Study the drawing (mm; zero at the part's minimum x, y, z) and answer. Coordinates: 2 decimals unless noted, no trailing zeros. Order: outer loops, then holes, each group sorted by start corner. A loop starts at its lowest first (then second) coordinate and runs counter-clockwise, first axis right, second up. Notation, with made-up numbers: M 40.5,65 L 63.5,65 A29 cw 63.5,94 Z; hole C 11,5 d5. An arc over 180 degrees is marked long. One line per item, written item: value. Start each with the question number.
Q1. The part is cut by section D-D on x = 6.5. Give the vertices of the cut face in (y, z), then the cut area to 3 significant figures.
Q2. The part is cut by section C-C on y = 26. Give the vertices of the cut face in (x, z), then the cut area to 3 significant figures.
Q3. The part is cut by section A-A on x = 25.8. Give the vertices of the cut face in (y, z).
Q4. Each of these flat-tipped pins is pushed along its axis until it touches: pin 1 Ø0.6 at (x, z) = (13.5, 2) entering from +Y; pin 2 Ø1.8 at (x, y) = (2, 2) entering from -Z; pin 3 Ø0.6 at (y, z) = (10, 2.5) entering from +X; pin 4 Ø3 at (x, y) = (25.8, 2) entering from +Z. Where does it stop, or does it pass through?
Q5. The part is cut by section B-B on z = 0.9. Give the vertices of the cut face in (x, y).
Q6. Straight lines are drawn through the part: line 1 along Y through (x, z) = (25.8, 0.8); line 2 along X through (y, z) = (12, 1.45); line 3 along Y through (x, z) = (26.25, 1.35). For each, find the intervals that lie inside material, in ascending order. Write a range as [from, to].
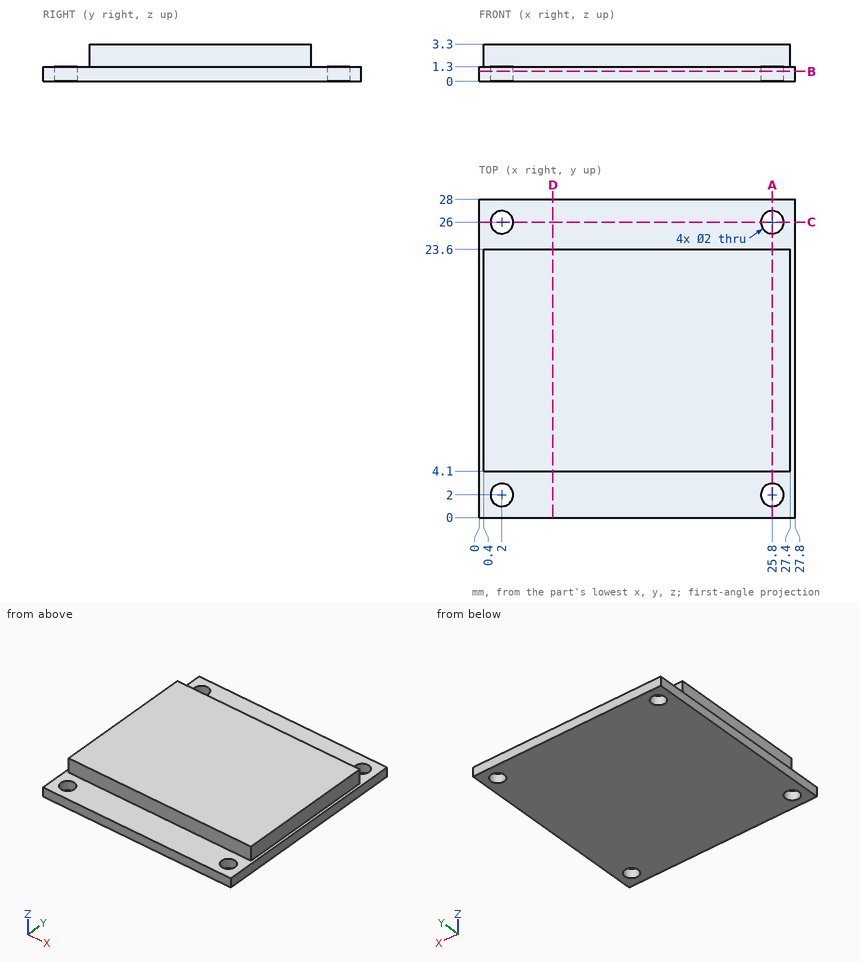
Output:
1. outline: M 0,0 L 28,0 L 28,1.3 L 23.6,1.3 L 23.6,3.3 L 4.1,3.3 L 4.1,1.3 L 0,1.3 Z
1. area: 75.4 mm^2
2. outline: M 0,0 L 1,0 L 1,1.3 L 0,1.3 Z; M 3,0 L 24.8,0 L 24.8,1.3 L 3,1.3 Z; M 26.8,0 L 27.8,0 L 27.8,1.3 L 26.8,1.3 Z
2. area: 30.9 mm^2
3. outline: M 0,0 L 1,0 L 1,1.3 L 0,1.3 Z; M 3,0 L 25,0 L 25,1.3 L 23.6,1.3 L 23.6,3.3 L 4.1,3.3 L 4.1,1.3 L 3,1.3 Z; M 27,0 L 28,0 L 28,1.3 L 27,1.3 Z
4. pin 1: stops at y = 23.6
4. pin 2: passes through
4. pin 3: stops at x = 27.4
4. pin 4: stops at z = 1.3
5. outline: M 0,0 L 27.8,0 L 27.8,28 L 0,28 Z; hole C 2,2 d2; hole C 2,26 d2; hole C 25.8,2 d2; hole C 25.8,26 d2
6. line 1: y = [0, 1], [3, 25], [27, 28]
6. line 2: x = [0.4, 27.4]
6. line 3: y = [4.1, 23.6]
